Design review of the part built by this model. Coordinates are the model's own, in mm. A direction names the side the tool comes from. Give positions to 0.01 mm unless a question says otherwise; leave off trailing zeros. Write each loop counter-clockwise with the first axis right and the second up, starting at its lowest first coordinate (ties: lowest second). Pieces come first, ordered by that corner, then holes.
Autodesk Inventor part; units mm, degrees
ref_plane "YZ Plane" through (0, 0, 0) normal (1, 0, 0) x (0, 1, 0)
ref_plane "XZ Plane" through (0, 0, 0) normal (0, 1, 0) x (-1, 0, 0)
ref_plane "XY Plane" through (0, 0, 0) normal (0, 0, 1) x (1, 0, 0)
sketch "Sketch1" plane through (0, 0, 0) normal (0, 0, 1) x (1, 0, 0)
  line L0 (-30, 5) -> (30, 5)
  line L1 (30, 5) -> (30, -5)
  line L2 (30, -5) -> (-30, -5)
  line L3 (-30, -5) -> (-30, 5)
  line L4 (-10, 35) -> (10, 35)
  line L5 (10, 35) -> (10, 5)
  line L6 (10, 5) -> (-10, 5)
  line L7 (-10, 5) -> (-10, 35)
  point P0 (0, 0)
  point P1 (0, 5)
  point P2 (-30, 0)
  point P3 (0, 5)
  dimension "d0" = 10
  dimension "d1" = 60
  dimension "d2" = 30
  dimension "d3" = 20
extrude "Extrusion1" add sketch "Sketch1" along normal blind 15
sketch "Sketch2" plane through (-30, 5, 0) normal (0, 1, 0) x (1, 0, 0)
  line L0 (30, -53.7244) -> (30, -44.0936) construction
  line L1 (40, -15) -> (20, -15) construction
  line L2 (0, 0) -> (0, -15)
  point P0 (30, 0)
  point P1 (55, -7.5)
  point P2 (5, -7.5)
  point P3 (30, -48.909)
  point P4 (30, -15)
  point P5 (0, -7.5)
  dimension "d6" = 50
hole "Hole1" at (25, 5, 7.5) at (-25, 5, 7.5) direction (0, -1, 0) diameter 5 end through all
sketch "Sketch3" plane through (0, 0, 15) normal (0, 0, 1) x (1, 0, 0)
  line L0 (-10, 35) -> (10, 35)
  line L1 (10, 35) -> (10, 15)
  line L2 (10, 15) -> (-10, 15)
  line L3 (-10, 15) -> (-10, 35)
  line L4 (10, 35) -> (-10, 35)
  line L5 (10, 5) -> (10, 35)
  line L6 (-10, 35) -> (-10, 5)
  line L7 (-10, 20) -> (-7, 20)
  line L8 (-7, 20) -> (-7, 15)
  line L9 (-7, 15) -> (-10, 15)
  line L10 (-10, 15) -> (-10, 20)
  line L11 (7, 20) -> (10, 20)
  line L12 (10, 20) -> (10, 15)
  line L13 (10, 15) -> (7, 15)
  line L14 (7, 15) -> (7, 20)
  line L15 (10, 5) -> (10, 35)
  point P0 (0, 0)
  point P1 (-10, 20)
  dimension "d14" = 20
  dimension "d15" = 3
  dimension "d16" = 5
extrude "Extrusion2" add sketch "Sketch3" along normal blind 35 contours L0 L1 L11 L14 L2 L8 L7 L3
sketch "Sketch4" plane through (-10, 5, 0) normal (-1, 0, 0) x (0, 0, 1)
  line L0 (50, 30) -> (50, 15)
  line L1 (15, 15) -> (15, 0)
  point P0 (0, -5)
  point P1 (25, 22.5)
  point P2 (50, 22.5)
  dimension "d27" = 25
hole "Hole2" at (-10, 27.5, 25) direction (1, 0, 0) diameter 5 end through all counterbore diameter 9 counterbore depth 5
properties part number "0008-10-054 Suport doking"
(1) Consider section A-A, the plane z = 7.5. Give the boundary of the cut face in (x, y), then the cut area to 3 significant figures.
Resolved:
outline: (-30, -5) - (-27.5, -5) - (-27.5, 5) - (-30, 5) - close; (-22.5, -5) - (22.5, -5) - (22.5, 5) - (10, 5) - (10, 35) - (-10, 35) - (-10, 5) - (-22.5, 5) - close; (27.5, -5) - (30, -5) - (30, 5) - (27.5, 5) - close
area: 1,100 mm2
(2) Consider section B-B, the plane x = 25. Give the boundary of the cut face in (y, z).
Resolved:
outline: (-5, 0) - (5, 0) - (5, 5) - (-5, 5) - close; (-5, 10) - (5, 10) - (5, 15) - (-5, 15) - close
(3) Mouldability with a two-part tool opening along Z and no side actions: class faces 1 (the face through (-7.465, 27.302, 20.504)), 2 (the face through (23, 0, 9)), 3 (the face through (20, 5, 7)), 4 (the face through (0, 11, 0)) as pulls with the +Z half, pulls with the -Z half, needs draft (parallel to the pull), parting line crosses it, or undercut.
Resolved:
face 1: undercut
face 2: undercut
face 3: needs draft
face 4: pulls with the -Z half
(4) To check wall thickness, follow L1, parallel to Z at x = -25, y = -2.5; L2, parallel to Y at x = -8, z = 25; L3, parallel to Z at x = -7.9, y = 27.5. State the ranges of each line that lie inside material, in increasing order.
Resolved:
L1: z = 0 to 5, 10 to 15
L2: y = 20 to 23, 32 to 35
L3: z = 0 to 20.5, 29.5 to 50
(5) Consider section D-D, the plane z = 45. Give the boundary of the cut face in (x, y), then the cut area to 3 significant figures.
Resolved:
outline: (-10, 20) - (-7, 20) - (-7, 15) - (7, 15) - (7, 20) - (10, 20) - (10, 35) - (-10, 35) - close
area: 370 mm2
(6) Clearance check with flat-ended pins moving along their axes: P1, Ø24, axis at y = 22.5, z = 30, coming from the +X side; P2, Ø12, axis at y = 14, z = 7.5, coming from the -X side; P3, Ø2.5, axis at x = -9, z = 35, coming from the -Y side. State where each tip first meets the part, or that it passes through.
Resolved:
P1: stops at x = 10
P2: stops at x = -10
P3: stops at y = 20
(7) Consider section C-C, the plane z = 25. Give the boundary of the cut face in (x, y).
Resolved:
outline: (-10, 20) - (-7, 20) - (-7, 15) - (7, 15) - (7, 20) - (10, 20) - (10, 25) - (-5, 25) - (-5, 23) - (-10, 23) - close; (-10, 32) - (-5, 32) - (-5, 30) - (10, 30) - (10, 35) - (-10, 35) - close
(8) Tool access review of faces 5 (the face through (-7, 18, 32)), 6 (the face through (7, 17, 32)), 7 (the face through (0, 15, 32)): name each direction out of +Z, -Z, +X, -X, +Y, -Y from which nothing blocks a thin tool from reaching the whole face with its end or side.
Resolved:
face 5: +Z, -X, -Y
face 6: +Z, +X, -Y
face 7: +Z, +X, -X, -Y
